The listing builds one solid part. Answer for the finished solid, in the listing's coordinates (mm). A direction names the side the tool comes from. Give positions to 0.01 mm unless a question says otherwise; leave off trailing zeros. Write each loop counter-clockwise with the first axis right and the second up, starting at its lowest first coordinate (ties: lowest second). Pieces come first, ordered by that corner, then holes. Notation, with made-up numbers: (23, -7.5) - (32, -7.5) arc R8 ccw to (32, 5.5) - close; hole circle Ø6 at (50.5, 10.25). An arc over 180 degrees is marked (long way). Answer as CSV lines item,"result". Start each with the question number.
(1) For faces 4 (the face through (145, -145, 2)), 5 (the face through (157.89, -107.46, 2.46)), 6 (the face through (169, -89, 5)), determine the directions among +Z, -Z, +X, -X, +Y, -Y from which every point of the face is accessible in a straight line to the end or side of a thin tool.
(2) Find section A-A (y = -151). Write down the section's boundary in (x, z).
(3) Straight lines are drawn through the part: probe 1 along X at (y, z) = (-158, 1.9); probe 2 along X at (y, z) = (-112, 3.8); probe 3 along Y at (x, z) = (124.5, 2.8). For each, find the intervals that lie inside material, in ascending order.
(4) Find section B-B (z = 0.9). Write down the section's boundary in (x, y).
(5) For a pull along X with two mould halves and no side action, classify faces 1 (the face through (0, -89, 2)), 2 (the face through (67, -180, 2)), 3 (the face through (146, -178, 3)) as pulls with the +X half, pulls with the -X half, needs draft (parallel to the pull), parting line crosses it, or undercut.
(6) Find section C-C (y = -85). Write down the section's boundary in (x, z).
from build123d import *

# Parameters (mm, degrees)
F1_DEPTH = 5
F2_R     = 5
F3_R     = 1


with BuildPart() as f1:
    # F0 (on Top) → F1 (new body)
    with BuildSketch(Plane.XY):
        with BuildLine():
            Line((140, 0), (0, 0))
            Line((0, 0), (0, -95.548943))
            Line((0, -95.548943), (115.623593, -95.548943))
            ThreePointArc((115.623593, -95.548943), (120.458716, -74.40711), (140, -65))
            Line((140, -65), (140, 0))
        make_face()
        with BuildLine():
            Line((280, 0), (140, 0))
            Line((140, 0), (140, -65))
            ThreePointArc((140, -65), (157.67767, -72.32233), (165, -90))
            ThreePointArc((165, -90), (164.843613, -92.791936), (164.376407, -95.548943))
            Line((164.376407, -95.548943), (280, -95.548943))
            Line((280, -95.548943), (280, 0))
        make_face()
        with BuildLine():
            Line((280, -180), (280, -95.548943))
            Line((280, -95.548943), (164.376407, -95.548943))
            ThreePointArc((164.376407, -95.548943), (157.478004, -107.875105), (145, -114.494897))
            Line((145, -114.494897), (145, -180))
            Line((145, -180), (280, -180))
        make_face()
        with BuildLine():
            Line((115.623593, -95.548943), (0, -95.548943))
            Line((0, -95.548943), (0, -180))
            Line((0, -180), (135, -180))
            Line((135, -180), (135, -114.494897))
            ThreePointArc((135, -114.494897), (122.521996, -107.875105), (115.623593, -95.548943))
        make_face()
    extrude(amount=F1_DEPTH)

    # F2
    f2_edges = [f1.edges().sort_by_distance(p)[0] for p in [
        (135, -180, 2.5),
        (145, -180, 2.5),
        (280, -180, 2.5),
        (0, -180, 2.5),
        (280, 0, 2.5),
        (0, 0, 2.5),
    ]]
    fillet(f2_edges, radius=F2_R)

    # F3
    f3_edges = [f1.edges().sort_by_distance(p)[0] for p in [
        (135, -114.494897, 2.5),
        (145, -114.494897, 2.5),
    ]]
    fillet(f3_edges, radius=F3_R)


solid = f1.part
Result set:
1,face 4,"+Z, -Z, -Y"
1,face 5,"+Z, -Z"
1,face 6,"+Z, +X, -X, +Y, -Y"
2,outline,"(0, 0) - (135, 0) - (135, 5) - (0, 5) - close; (145, 0) - (280, 0) - (280, 5) - (145, 5) - close"
3,probe 1,"0 to 135, 145 to 280"
3,probe 2,"0 to 128.13, 151.87 to 280"
3,probe 3,"-180 to -109.62, -70.38 to 0"
4,outline,"(0, -175) arc R5 ccw to (5, -180) - (130, -180) arc R5 ccw to (135, -175) - (135, -115.3) arc R1 ccw to (134.23, -114.33) arc R25 cw to (115.62, -95.55) arc R25 cw to (140, -65) arc R25 cw to (165, -90) arc R25 cw to (164.38, -95.55) arc R25 cw to (145.77, -114.33) arc R1 ccw to (145, -115.3) - (145, -175) arc R5 ccw to (150, -180) - (275, -180) arc R5 ccw to (280, -175) - (280, -5) arc R5 ccw to (275, 0) - (5, 0) arc R5 ccw to (0, -5) - close"
5,face 1,"pulls with the -X half"
5,face 2,"needs draft"
5,face 3,"undercut"
6,outline,"(0, 0) - (115.51, 0) - (115.51, 5) - (0, 5) - close; (164.49, 0) - (280, 0) - (280, 5) - (164.49, 5) - close"
